For this review, take the finished solid that the model builds, in its own axes (mm). A direction names the side the tool comes from. Coordinates: 2 decimals unless noted, no trailing zeros.
1. To check wall thickness, follow probe 1 along Z at (x, y) = (-12, 1.6); probe 2 along X at (y, z) = (2.25, -8.5) (3 decimals); probe 3 along Z at (x, y) = (0, 1.5). State the ranges of each line that lie inside material, in increasing order.
2. Mouldability with a two-part tool opening along Z and no side actions: class faces 3 (the face through (-15.52, 1.63, 15.42)), 4 (the face through (-2, 3.302, 5)) as pulls with the +Z half, pulls with the -Z half, needs draft (parallel to the pull), parting line crosses it, or undercut.
3. Take a section at A-A, the plane z = -14.5. Count the separate pieces of the cut face and the enclosed holes in it, then the cut area to 3 significant figures.
4. Machinability: for faces 1 (the face through (-9.9, 1.63, 19.43)), 2 (the face through (-2, 0, 5)), which of the approach directions +Z, -Z, +X, -X, +Y, -Y give a long, thin tool a straight path to every point of the face, cutting with its end or side? Answer none if there is none.
5. Clearance check with flat-ended pins moving along their axes: P1, Ø4, axis at x = -19.5, z = -21.5, coming from the +Y side; P2, Ø1, axis at x = -9.5, y = 1, coming from the +Z side; P3, Ø1, axis at y = 2.5, z = -14, coming from the -X side; P4, Ø3, axis at x = 0, z = 0, coming from the -Y side. State where each tip first meets the part, or that it passes through.
```python
from build123d import *

# Parameters (mm, degrees)
SKETCH1_R           = 26.9875
BOSS_EXTRUDE1_DEPTH = 3.302
FILLET1_R           = 3.81
SKETCH2_R           = 1.5875


with BuildPart() as part:
    # Sketch1 → Boss-Extrude1 (new body)
    with BuildSketch(Plane(origin=(0, 0, 0), x_dir=(1, 0, 0), z_dir=(0, 1, 0))):
        with Locations(Location((0, 0, 0), (0, 0, 90))):
            Circle(SKETCH1_R)
        with BuildLine():
            Line((-1.905, 23.099079662), (-1.905, 4.709286039))
            ThreePointArc((-1.905, 4.709286039), (-2.985949082, 4.109806331), (-3.8901198, 3.267012081))
            Line((-3.8901198, 3.267012081), (-21.379852859, 8.949770834))
            ThreePointArc((-21.379852859, 8.949770834), (-13.623392685, 18.750991387), (-1.905, 23.099079662))
        make_face(mode=Mode.SUBTRACT)
        with BuildLine():
            Line((1.905, 23.099079662), (1.905, 4.709286039))
            ThreePointArc((1.905, 4.709286039), (2.985949082, 4.109806331), (3.8901198, 3.267012081))
            Line((3.8901198, 3.267012081), (21.379852859, 8.949770834))
            ThreePointArc((21.379852859, 8.949770834), (13.623392685, 18.750991387), (1.905, 23.099079662))
        make_face(mode=Mode.SUBTRACT)
        with BuildLine():
            Line((-22.557207608, 5.326245507), (-5.067474549, -0.356513246))
            ThreePointArc((-5.067474549, -0.356513246), (-4.831367103, -1.569806331), (-4.309226257, -2.690161532))
            Line((-4.309226257, -2.690161532), (-15.118475741, -17.567817096))
            ThreePointArc((-15.118475741, -17.567817096), (-22.043112406, -7.162241387), (-22.557207608, 5.326245507))
        make_face(mode=Mode.SUBTRACT)
        with BuildLine():
            Line((-1.226871508, -4.929623343), (-12.036120993, -19.807278907))
            ThreePointArc((-12.036120993, -19.807278907), (0, -23.1775), (12.036120993, -19.807278907))
            Line((12.036120993, -19.807278907), (1.226871508, -4.929623343))
            ThreePointArc((1.226871508, -4.929623343), (0, -5.08), (-1.226871508, -4.929623343))
        make_face(mode=Mode.SUBTRACT)
        with BuildLine():
            Line((22.557207608, 5.326245507), (5.067474549, -0.356513246))
            ThreePointArc((5.067474549, -0.356513246), (4.831367103, -1.569806331), (4.309226257, -2.690161532))
            Line((4.309226257, -2.690161532), (15.118475741, -17.567817096))
            ThreePointArc((15.118475741, -17.567817096), (22.043112406, -7.162241387), (22.557207608, 5.326245507))
        make_face(mode=Mode.SUBTRACT)
        with BuildLine():
            Line((-1.226374532, 1.253998), (1.226374532, 1.253998))
            ThreePointArc((1.226374532, 1.253998), (0, -1.753997), (-1.226374532, 1.253998))
        make_face(mode=Mode.SUBTRACT)
    extrude(amount=BOSS_EXTRUDE1_DEPTH)

    # Fillet1
    # the kernel refuses this fillet: 3.81 mm, written as the material it adds along each edge
    with BuildSketch(Plane(origin=(-22.557207608, 0, -5.326245507), x_dir=(0.9510565162951546, 0, 0.3090169943749439), z_dir=(0, 1, 0)), Plane(origin=(-1.905, 0, -23.099079662), x_dir=(0, 0, 1), z_dir=(0, 1, 0))) as fillet1_piece_1:
        with BuildLine():
            CenterArc((4.593976819, -3.81), FILLET1_R, 90, 107.162452548)
            ThreePointArc((0.953628718, -4.934262295), (0.342682242, -2.493054423), (0, 0))
            Line((0, 0), (4.593976819, 0))
        make_face()
    extrude(amount=3.302)
    with BuildSketch(Plane(origin=(-5.067474549, 0, 0.356513246), x_dir=(-0.9510565162951546, 0, -0.3090169943749442), z_dir=(0, 1, 0)), Plane(origin=(-1.226871508, 0, 4.929623343), x_dir=(-0.5877852522924791, 0, 0.8090169943749429), z_dir=(0, 1, 0)), Plane(origin=(4.309226257, 0, 2.690161532), x_dir=(0.5877852522924685, 0, 0.8090169943749509), z_dir=(0, 1, 0)), Plane(origin=(-1.905, 0, -4.709286039), x_dir=(0, 0, -1), z_dir=(0, 1, 0))) as fillet1_piece_2:
        with BuildLine():
            CenterArc((2.100330323, 3.81), FILLET1_R, 220.005200885, 49.994799115)
            ThreePointArc((-0.818076689, 1.360714286), (-0.355550163, 0.712514837), (0, 0))
            Line((0, 0), (2.100330323, 0))
        make_face()
    extrude(amount=3.302)
    with BuildSketch(Plane(origin=(-4.309226257, 0, 2.690161532), x_dir=(-0.3904940341583853, 0, -0.9206054579931132), z_dir=(0, 1, 0)), Plane(origin=(1.226871508, 0, 4.929623343), x_dir=(-0.9962171125182067, 0, 0.08689916412651309), z_dir=(0, 1, 0)), Plane(origin=(5.067474549, 0, 0.356513246), x_dir=(-0.22520200155214, 0, 0.9743120950172537), z_dir=(0, 1, 0)), Plane(origin=(1.905, 0, -4.709286039), x_dir=(0.8570346212244796, 0, 0.5152588262442601), z_dir=(0, 1, 0)), Plane(origin=(-3.8901198, 0, -3.267012081), x_dir=(0.7548785270042563, 0, -0.6558646273949256), z_dir=(0, 1, 0))) as fillet1_piece_3:
        with BuildLine():
            CenterArc((2.18308817, 3.763191931), FILLET1_R, 211.014756861, 49.994799115)
            Line((-1.082213737, 1.800055803), (0, 0))
            ThreePointArc((0, 0), (0.793850244, 0.062410759), (1.587700487, 0))
        make_face()
    extrude(amount=3.302)
    with BuildSketch(Plane(origin=(-15.118475741, 0, 17.567817096), x_dir=(0.5877852522924796, 0, -0.8090169943749426), z_dir=(0, 1, 0)), Plane(origin=(-21.379852859, 0, -8.949770834), x_dir=(0.9510565162951546, 0, 0.3090169943749444), z_dir=(0, 1, 0)), Plane(origin=(1.905, 0, -23.099079662), x_dir=(0, 0, 1), z_dir=(0, 1, 0))) as fillet1_piece_4:
        with BuildLine():
            CenterArc((4.593976819, 3.81), FILLET1_R, 162.837547452, 107.162452548)
            ThreePointArc((0.953628718, 4.934262295), (0.342682242, 2.493054423), (0, 0))
            Line((0, 0), (4.593976819, 0))
        make_face()
    extrude(amount=3.302)
    with BuildSketch(Plane(origin=(12.036120993, 0, 19.807278907), x_dir=(-0.9058536844822791, 0, 0.42359072500454903), z_dir=(0, 1, 0)), Plane(origin=(22.557207608, 0, -5.326245507), x_dir=(0.1229345363355818, 0, 0.9924147821228559), z_dir=(0, 1, 0))) as fillet1_piece_5:
        with BuildLine():
            CenterArc((4.612509297, -3.78754287), FILLET1_R, 83.776053996, 107.162452548)
            Line((0.871731639, -4.510510721), (0, 0))
            ThreePointArc((0, 0), (2.512784916, 0.136614205), (5.025569831, 0))
        make_face()
    extrude(amount=3.302)
    with BuildSketch(Plane(origin=(-12.036120993, 0, 19.807278907), x_dir=(0.9058536844822742, 0, 0.42359072500455974), z_dir=(0, 1, 0)), Plane(origin=(15.118475741, 0, 17.567817096), x_dir=(0.6827829021799576, 0, -0.7306213167508284), z_dir=(0, 1, 0)), Plane(origin=(21.379852859, 0, -8.949770834), x_dir=(-0.4838706439977688, 0, -0.8751395316617714), z_dir=(0, 1, 0))) as fillet1_piece_6:
        with BuildLine():
            CenterArc((4.612509297, 3.78754287), FILLET1_R, 169.061493455, 107.162452548)
            Line((0.871731639, 4.510510721), (0, 0))
            ThreePointArc((0, 0), (2.512784916, -0.136614205), (5.025569831, 0))
        make_face()
    extrude(amount=3.302)
    with BuildSketch(Plane(origin=(3.8901198, 0, -3.267012081), x_dir=(-0.7548785270042564, 0, -0.6558646273949251), z_dir=(0, 1, 0))) as fillet1_piece_7:
        with BuildLine():
            CenterArc((2.18308817, -3.763191931), FILLET1_R, 98.990444024, 49.994799115)
            Line((-1.082213737, -1.800055803), (0, 0))
            ThreePointArc((0, 0), (0.793850244, -0.062410759), (1.587700487, 0))
        make_face()
    extrude(amount=3.302)

    # Cut-Sweep1: sweep along a curve in space
    with BuildLine() as cut_sweep1_path:
        ThreePointArc((0, 0, 26.9875), (19.083044257, 0, 19.083044257), (26.9875, 0, 0))
        ThreePointArc((26.9875, 0, 0), (19.083044257, 0, -19.083044257), (0, 0, -26.9875))
        ThreePointArc((0, 0, -26.9875), (-19.083044257, 0, -19.083044257), (-26.9875, 0, 0))
        ThreePointArc((-26.9875, 0, 0), (-19.083044257, 0, 19.083044257), (0, 0, 26.9875))
    # Sketch2 → Cut-Sweep1 (sweep, cut)
    with BuildSketch(Plane(origin=(0, 0, 0), x_dir=(0, 0, -1), z_dir=(1, 0, 0))):
        with Locations((26.9875, 1.651)):
            Circle(SKETCH2_R)
    sweep(path=cut_sweep1_path.line, mode=Mode.SUBTRACT)


solid = part.part
```
Results list:
1. probe 1: z = -22.39 to -19.83, -5.9 to -1.9, 13.28 to 22.39
1. probe 2: x = -24.06 to -18.567, -1.905 to 1.905, 18.567 to 24.06
1. probe 3: z = -25.41 to -1.25, 1.75 to 5.11, 23.18 to 25.41
2. face 3: undercut
2. face 4: needs draft
3. separate pieces: 3
3. enclosed holes: 0
3. area: 34.0 mm2
4. face 1: +Y, -Y
4. face 2: +Z, -Z, +X, -X, -Y
5. P1: passes through
5. P2: stops at z = 24.12
5. P3: stops at x = -22.14
5. P4: stops at y = 0
